from build123d import *

# Parameters (mm, degrees)
SKETCH1_R           = 29.5
BOSS_EXTRUDE1_DEPTH = 4.5
CUT_EXTRUDE1_DEPTH  = 42.961291687
CUT_EXTRUDE2_DEPTH  = 42.961291687


with BuildPart() as part:
    # Sketch1 → Boss-Extrude1 (new body)
    with BuildSketch(Plane(origin=(0, 0, 0), x_dir=(1, 0, 0), z_dir=(0, 1, 0))):
        with Locations(Location((0, 0, 0), (0, 0, 270))):
            Circle(SKETCH1_R)
    extrude(amount=BOSS_EXTRUDE1_DEPTH)

    # Sketch2 → Cut-Extrude1 (cut, through all)
    with BuildSketch(Plane(origin=(0, 4.5, 0), x_dir=(1, 0, 0), z_dir=(0, 1, 0))):
        with BuildLine():
            Line((-8.5, -22.5), (8.5, -22.5))
            ThreePointArc((8.5, -22.5), (10.267766953, -21.767766953), (11, -20))
            Line((11, -20), (11, 20))
            ThreePointArc((11, 20), (10.267766953, 21.767766953), (8.5, 22.5))
            Line((8.5, 22.5), (-8.5, 22.5))
            ThreePointArc((-8.5, 22.5), (-10.267766953, 21.767766953), (-11, 20))
            Line((-11, 20), (-11, -20))
            ThreePointArc((-11, -20), (-10.267766953, -21.767766953), (-8.5, -22.5))
        make_face()
    extrude(amount=-CUT_EXTRUDE1_DEPTH, mode=Mode.SUBTRACT)

    # Sketch3 → Cut-Extrude2 (cut, through all)
    with BuildSketch(Plane(origin=(0, 4.5, 0), x_dir=(1, 0, 0), z_dir=(0, 1, 0))):
        with BuildLine():
            ThreePointArc((-27, 9), (-26.121320344, 11.121320344), (-24, 12))
            Line((-24, 12), (-19.5, 12))
            ThreePointArc((-19.5, 12), (-17.378679656, 11.121320344), (-16.5, 9))
            Line((-16.5, 9), (-16.5, 0))
            Line((-16.5, 0), (-16.5, -9))
            ThreePointArc((-16.5, -9), (-17.378679656, -11.121320344), (-19.5, -12))
            Line((-19.5, -12), (-24, -12))
            ThreePointArc((-24, -12), (-26.121320344, -11.121320344), (-27, -9))
            Line((-27, -9), (-27, 9))
        make_face()
        with BuildLine():
            Line((16.5, -9), (16.5, 0))
            Line((16.5, 0), (16.5, 9))
            ThreePointArc((16.5, 9), (17.378679656, 11.121320344), (19.5, 12))
            Line((19.5, 12), (24, 12))
            ThreePointArc((24, 12), (26.121320344, 11.121320344), (27, 9))
            Line((27, 9), (27, -9))
            ThreePointArc((27, -9), (26.121320344, -11.121320344), (24, -12))
            Line((24, -12), (19.5, -12))
            ThreePointArc((19.5, -12), (17.378679656, -11.121320344), (16.5, -9))
        make_face()
    extrude(amount=-CUT_EXTRUDE2_DEPTH, mode=Mode.SUBTRACT)

    # Sketch4 → Revolve1 (revolve)
    with BuildSketch(Plane(origin=(0, 0, 0), x_dir=(0, 0, -1), z_dir=(1, 0, 0))):
        with BuildLine():
            ThreePointArc((31.75, 2.25), (31.090990258, 3.840990258), (29.5, 4.5))
            Line((29.5, 4.5), (29.5, 0))
            ThreePointArc((29.5, 0), (31.090990258, 0.659009742), (31.75, 2.25))
        make_face()
    revolve(axis=Axis((0, 0, 0), (0, 1, 0)))


solid = part.part
Could you check a few things on this model? Use its own coordinates, in mm. A direction names the side the tool comes from. Round coordinates to 2 decimals unless told otherwise and drop trailing zeros. Write each loop counter-clockwise with the first axis right and the second up, starting at its lowest first coordinate (ties: lowest second). Pieces come first, ordered by that corner, then holes. Notation, with made-up numbers: (0.5, 68) - (59.5, 68) arc R23 cw to (59.5, 82) - close; hole circle Ø11 at (-29, -5). An arc over 180 degrees is marked (long way). Put each result on its own line as item: value. Start each with the question number.
(1) I need wall thicknesses on probe 1 along X at (y, z) = (1.9, -11.5); probe 2 along X at (y, z) = (1.6, -5); probe 3 along Z at (x, y) = (-17.5, 0.85). Which ranges of each line are inside material? Lowest first, please.
(2) Will these pins go through, and if not, where does the flat tip stop? pin 1 (2 mm diameter, centred on x = 10.5, y = 3.5, fed in from +Z); pin 2 (1 mm diameter, centred on x = -25, y = 1.5, fed in from +Z); pin 3 (1 mm diameter, centred on x = 19, y = 2.5, fed in from +Z).
(3) I want a section at B-B, the plane z = -7. Give the number of separate pieces and of enclosed holes in the cut face, plus the area to 3 significant figures.
(4) For faces 1 (the cylindrical face through (-17.36, 2.28, 11.1)), 2 (the flat face through (-13, 4.5, 0)), which set-ups out of +Z, -Z, +X, -X, +Y, -Y let a thin tool reach every point of the face, with its end or its side?
(5) I want a section at A-A, the plane y = 1.5. Please give me the cut outline in (x, z).
(6) Thinking about a two-plate mould opening in Z: for faces 3 (the cylindrical face through (26.1, 2.28, -11.14)), 4 (the cylindrical face through (26.14, 2.28, 11.1)), 5 (the flat face through (-13, 0, 0)), which applies, released by +Z, released by -Z, zero draft, split by the parting line, or undercut?
Here are the results:
1. probe 1: x = -29.56 to -25.66, -17.84 to -11, 11 to 17.84, 25.66 to 29.56
1. probe 2: x = -31.26 to -27, -16.5 to -11, 11 to 16.5, 27 to 31.26
1. probe 3: z = -25.9 to -11.24, 11.24 to 25.9
2. pin 1: stops at z = 30.13
2. pin 2: stops at z = 20.04
2. pin 3: stops at z = 25.79
3. separate pieces: 4
3. enclosed holes: 0
3. area: 80.8 mm^2
4. face 1: +Y, -Y
4. face 2: +Z, -Z, +X, -X, +Y
5. outline: circle Ø63.24 at (0, 0); hole (-27, -9) arc R3 ccw to (-24, -12) - (-19.5, -12) arc R3 ccw to (-16.5, -9) - (-16.5, 9) arc R3 ccw to (-19.5, 12) - (-24, 12) arc R3 ccw to (-27, 9) - close; hole (-11, -20) arc R2.5 ccw to (-8.5, -22.5) - (8.5, -22.5) arc R2.5 ccw to (11, -20) - (11, 20) arc R2.5 ccw to (8.5, 22.5) - (-8.5, 22.5) arc R2.5 ccw to (-11, 20) - close; hole (16.5, -9) arc R3 ccw to (19.5, -12) - (24, -12) arc R3 ccw to (27, -9) - (27, 9) arc R3 ccw to (24, 12) - (19.5, 12) arc R3 ccw to (16.5, 9) - close
6. face 3: undercut
6. face 4: undercut
6. face 5: zero draft
